Work out the finished part from the listing and answer in its coordinate system (mm). Face numbers are marked on the shaded views. A direction names the side the tool comes from. Round coordinates to 2 decimals unless told otherwise and drop trailing zeros. Loops run counter-clockwise (first coordinate to the right, second up) from the corner with the lowest first, then second, coordinate; pieces in that order, holes last.
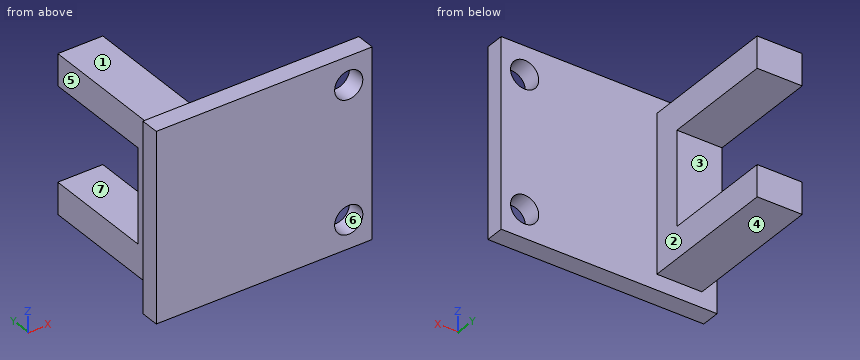
Autodesk Inventor part; units mm, degrees
ref_plane "YZ Plane" through (0, 0, 0) normal (1, 0, 0) x (0, 1, 0)
ref_plane "XZ Plane" through (0, 0, 0) normal (0, 1, 0) x (-1, 0, 0)
ref_plane "XY Plane" through (0, 0, 0) normal (0, 0, 1) x (1, 0, 0)
sketch "Sketch1" plane through (0, 0, 0) normal (0, 1, 0) x (-1, 0, 0)
  line L0 (11.5, 10) -> (-11.5, 10)
  line L1 (-11.5, 10) -> (-11.5, -10)
  line L2 (-11.5, -10) -> (11.5, -10)
  line L3 (11.5, -10) -> (11.5, 10)
  line L4 (11.5, 10) -> (-11.5, -10) construction
  line L5 (-11.5, 10) -> (11.5, -10) construction
  line L6 (-11.5, 0) -> (-11.5, -7)
  line L7 (-11.5, 0) -> (-11.5, 7)
  line L8 (-11.5, 7) -> (-9, 7)
  circle A0 centre (-9, 7) radius 1.5
  line L9 (-11.5, -7) -> (-9, -7)
  circle A1 centre (-9, -7) radius 1.5
  point P0 (0, 0)
  dimension "d0" = 23
  dimension "d1" = 20
  dimension "d2" = 7
  dimension "d3" = 7
  dimension "d4" = 2.5
  dimension "d5" = 3
  dimension "d6" = 3
extrude "Extrusion1" add sketch "Sketch1" along normal blind 2
sketch "Sketch2" plane through (0, 2, 0) normal (0, 1, 0) x (1, 0, 0)
  line L0 (-5.0848, -8.3507) -> (-9.8803, -8.3507)
  line L1 (-9.8803, -8.3507) -> (-9.8803, 8.3507)
  line L2 (-9.8803, 8.3507) -> (-5.0848, 8.3507)
  line L3 (-5.0848, 8.3507) -> (-5.0848, -8.3507)
  line L4 (-5.0848, -8.3507) -> (-9.8803, 8.3507) construction
  line L5 (-9.8803, -8.3507) -> (-5.0848, 8.3507) construction
  line L6 (-9.8803, 0) -> (-9.8803, 5)
  line L7 (-9.8803, 0) -> (-9.8803, -5)
  line L8 (-9.8803, -5) -> (-5.0848, -5)
  line L9 (-5.0848, -5) -> (-5.0848, -8.3507)
  line L10 (-5.0848, -8.3507) -> (-9.8803, -8.3507)
  line L11 (-9.8803, -8.3507) -> (-9.8803, -5)
  line L12 (-9.8803, 5) -> (-5.0848, 5)
  line L13 (-5.0848, 5) -> (-5.0848, 8.3507)
  line L14 (-5.0848, 8.3507) -> (-9.8803, 8.3507)
  line L15 (-9.8803, 8.3507) -> (-9.8803, 5)
  point P0 (0, 0)
  point P1 (-7.4826, 0)
  dimension "d9" = 5
  dimension "d10" = 5
extrude "Extrusion2" add sketch "Sketch2" along normal blind 15 contours L0 L1 L8 L3 | L12 L1 L2 L3
sketch "Sketch3" plane through (0, 2, 0) normal (0, 1, 0) x (1, 0, 0)
  line L0 (-5.0848, -8.3507) -> (-5.0848, -5)
  line L1 (-9.8803, 5) -> (-5.0848, 5)
  line L2 (-5.0848, -5) -> (-9.8803, -5)
  line L3 (-9.8803, -5) -> (-9.8803, 5)
  line L4 (-9.8803, 5) -> (-5.0848, 5)
  line L5 (-5.0848, 5) -> (-5.0848, -5)
  point P0 (0, 0)
extrude "Extrusion3" add sketch "Sketch3" along normal blind 3
ref_plane "Work Plane1" through (-5.0848, 17, 0) normal (0, 0, -1) x (-1, 0, 0)
ref_plane "Work Plane2" through (-7.4826, 2, -8.3507) normal (-1, 0, 0) x (0, 0, 1)
properties part number "lichtschrankenmodulmodell"
1. Which of the six approach directions +Z, -Z, +X, -X, +Y, -Y give full straight-line access (tool end or side, diameter ignored) to the marked faces 1, 2, 3 and 4?
Answer key:
face 1: +Z, +X, -X, +Y
face 2: +Z, -Z, +X, +Y
face 3: +X, -X, +Y
face 4: -Z, +X, -X, +Y
2. Find section A-A (x = 9). Write down the section's boundary in (y, z), then the cut area to 3 significant figures.
Answer key:
outline: (0, -10) - (2, -10) - (2, -8.5) - (0, -8.5) - close; (0, -5.5) - (2, -5.5) - (2, 5.5) - (0, 5.5) - close; (0, 8.5) - (2, 8.5) - (2, 10) - (0, 10) - close
area: 28.0 mm2
3. Find section C-C (y = 6). Write down the section's boundary in (x, z), then the cut area to 3 significant figures.
Answer key:
outline: (-9.88, -8.35) - (-5.08, -8.35) - (-5.08, -5) - (-9.88, -5) - close; (-9.88, 5) - (-5.08, 5) - (-5.08, 8.35) - (-9.88, 8.35) - close
area: 32.1 mm2
4. Determine the mould class of the marked faces 5, 6 and 7 for opening direction X: +X half, -X half, draft (parallel to the pull), parting line (faces both ways), or undercut.
Answer key:
face 5: -X half
face 6: undercut
face 7: draft
5. Given pin 1 (4.5 mm diameter, centred on y = 6, z = 0, fed in from +X); pin 2 (1.4 mm diameter, centred on x = -6.5, y = 9.5, fed in from +Z); pin 3 (5.5 mm diameter, centred on x = -7.5, y = 10, fed in from -Z), each flat-ended and moving along its own axis, determine where each tip first touches the part or whether it passes through.
Answer key:
pin 1: stops at x = -5.08
pin 2: stops at z = 8.35
pin 3: stops at z = -8.35
6. Consider probe 1 along Z at (x, y) = (9, 1.4); probe 2 along X at (y, z) = (0.7, 7); probe 3 along Z at (x, y) = (-9, 3.75). Determine where each line is inside the solid, lowest interval first.
Answer key:
probe 1: z = -10 to -8.5, -5.5 to 5.5, 8.5 to 10
probe 2: x = -11.5 to 7.5, 10.5 to 11.5
probe 3: z = -8.35 to 8.35
7. Find section B-B (z = -7). Write down the section's boundary in (x, y), then the cut area to 3 significant figures.
Answer key:
outline: (-11.5, 0) - (7.5, 0) - (7.5, 2) - (-5.08, 2) - (-5.08, 17) - (-9.88, 17) - (-9.88, 2) - (-11.5, 2) - close; (10.5, 0) - (11.5, 0) - (11.5, 2) - (10.5, 2) - close
area: 112 mm2
8. Find section D-D (x = -7.75). Write down the section's boundary in (y, z).
Answer key:
outline: (0, -10) - (2, -10) - (2, -8.35) - (17, -8.35) - (17, -5) - (5, -5) - (5, 5) - (17, 5) - (17, 8.35) - (2, 8.35) - (2, 10) - (0, 10) - close
